Geometry check sheet. Reference: the model listing, model coordinates, mm. Coordinates: 2 decimals unless noted, no trailing zeros. Write each loop counter-clockwise with the first axis right and the second up, starting at its lowest first coordinate (ties: lowest second). Pieces come first, ordered by that corner, then holes.
from build123d import *

# Parameters (mm, degrees)
SKETCH2_R           = 5
SKETCH2_R_2         = 10
BOSS_EXTRUDE1_DEPTH = 10
SCALE2_SCALE        = 0.2004


with BuildPart() as part:
    # Sketch2 → Boss-Extrude1 (new body)
    with BuildSketch(Plane(origin=(0, 0, 0), x_dir=(1, 0, 0), z_dir=(0, 1, 0))):
        with BuildLine():
            Line((-50, 20), (50, 20))
            ThreePointArc((50, 20), (70, 0), (50, -20))
            Line((50, -20), (-50, -20))
            ThreePointArc((-50, -20), (-70, 0), (-50, 20))
        make_face()
        with Locations(Location((50, 0, 0), (0, 0, 270))):
            Circle(SKETCH2_R, mode=Mode.SUBTRACT)
        with Locations(Location((-50, 0, 0), (0, 0, 270))):
            Circle(SKETCH2_R, mode=Mode.SUBTRACT)
        with Locations(Location((0, 0, 0), (0, 0, 270))):
            Circle(SKETCH2_R_2, mode=Mode.SUBTRACT)
    extrude(amount=BOSS_EXTRUDE1_DEPTH)


with BuildPart() as part_1:
    # Scale2: scaled about (0, 5, 0)
    add(part.part.scale(SCALE2_SCALE).moved(Location((0, 3.998, 0))))


solid = part_1.part
1. Draft check along X on faces 1 (the cylindrical face through (-14.027, 4.986, 0.088)), 2 (the flat face through (0, 5, -4.008)), 3 (the cylindrical face through (-1.22, 4.99, -1.59)). Enter one of: released by +X, released by -X, zero draft, split by the parting line, or undercut.
Computed values:
face 1: released by -X
face 2: zero draft
face 3: undercut
2. Thickness scan on line 1 along X through (y, z) = (5.05, 0); line 2 along X through (y, z) = (5.7, -0.5); line 3 along X through (y, z) = (5, -1.75). Record the ranges inside material, lowest first.
Computed values:
line 1: x = -14.03 to -11.02, -9.02 to -2, 2 to 9.02, 11.02 to 14.03
line 2: x = -14 to -10.89, -9.15 to -1.94, 1.94 to 9.15, 10.89 to 14
line 3: x = -13.63 to -0.98, 0.98 to 13.63
3. Sectioned sample at C-C, the plane y = 4.85. Record the boundary of the cut face in (x, z).
Computed values:
outline: (-10.02, -4.01) - (10.02, -4.01) arc R4.01 ccw to (10.02, 4.01) - (-10.02, 4.01) arc R4.01 ccw to start; hole circle Ø2 at (-10.02, 0); hole circle Ø4.01 at (0, 0); hole circle Ø2 at (10.02, 0)
4. Sectioned sample at A-A, the plane z = 0. Record the boundary of the cut face in (x, y), and give its area (3 significant figures).
Computed values:
outline: (-14.03, 4) - (-11.02, 4) - (-11.02, 6) - (-14.03, 6) - close; (-9.02, 4) - (-2, 4) - (-2, 6) - (-9.02, 6) - close; (2, 4) - (9.02, 4) - (9.02, 6) - (2, 6) - close; (11.02, 4) - (14.03, 4) - (14.03, 6) - (11.02, 6) - close
area: 40.2 mm2
5. Sectioned sample at B-B, the plane x = 0. Record the boundary of the cut face in (y, z).
Computed values:
outline: (4, -4.01) - (6, -4.01) - (6, -2) - (4, -2) - close; (4, 2) - (6, 2) - (6, 4.01) - (4, 4.01) - close
6. Sectioned sample at D-D, the plane z = 1.75. Record the boundary of the cut face in (x, y), and give its area (3 significant figures).
Computed values:
outline: (-13.63, 4) - (-0.98, 4) - (-0.98, 6) - (-13.63, 6) - close; (0.98, 4) - (13.63, 4) - (13.63, 6) - (0.98, 6) - close
area: 50.7 mm2
